from build123d import *

# Parameters (mm, degrees)
SKETCH1_W           = 111.125
SKETCH1_H           = 82.55
SKETCH1_R           = 4.7625
BOSS_EXTRUDE1_DEPTH = 6.35
SKETCH2_R           = 2.413
CUT_EXTRUDE1_DEPTH  = 12.7
SKETCH3_R           = 2.413
CUT_EXTRUDE2_DEPTH  = 12.7
SKETCH4_R           = 2.413
SKETCH4_W           = 22.225
SKETCH4_H           = 22.225
CUT_EXTRUDE3_DEPTH  = 7.62


with BuildPart() as part:
    # Sketch1 → Boss-Extrude1 (new body)
    with BuildSketch(Plane.XY):
        Rectangle(SKETCH1_W, SKETCH1_H)
        with Locations((0, 30.1625)):
            Circle(SKETCH1_R, mode=Mode.SUBTRACT)
        with Locations(Location((0, -30.1625, 0), (0, 0, 180))):
            Circle(SKETCH1_R, mode=Mode.SUBTRACT)
    extrude(amount=BOSS_EXTRUDE1_DEPTH)

    # Sketch2 → Cut-Extrude1 (cut)
    with BuildSketch(Plane(origin=(55.5625, 0, 0), x_dir=(0, 0, -1), z_dir=(1, 0, 0))):
        with Locations((-3.175, 20.6375)):
            Circle(SKETCH2_R)
        with Locations((-3.175, 0)):
            Circle(SKETCH2_R)
        with Locations((-3.175, -20.6375)):
            Circle(SKETCH2_R)
    cut_extrude1 = extrude(amount=-CUT_EXTRUDE1_DEPTH, mode=Mode.SUBTRACT)

    # Mirror1: Cut-Extrude1 across plane
    add(cut_extrude1.mirror(Plane(origin=(0, 0, 0), x_dir=(0, 0, 1), z_dir=(1, 0, 0))), mode=Mode.SUBTRACT)

    # Sketch3 → Cut-Extrude2 (cut)
    with BuildSketch(Plane(origin=(0, 41.275, 0), x_dir=(1, 0, 0), z_dir=(0, 1, 0))):
        with Locations(Location((0, -3.175, 0), (0, 0, 180))):
            Circle(SKETCH3_R)
    cut_extrude2 = extrude(amount=-CUT_EXTRUDE2_DEPTH, mode=Mode.SUBTRACT)

    # Mirror2: Cut-Extrude2 across plane
    add(cut_extrude2.mirror(Plane.ZX), mode=Mode.SUBTRACT)

    # Sketch4 → Cut-Extrude3 (cut)
    with BuildSketch(Plane.XY.offset(6.35)):
        with Locations((17.4625, 0)):
            Circle(SKETCH4_R)
        with Locations((-17.4625, 0)):
            Circle(SKETCH4_R)
        Rectangle(SKETCH4_W, SKETCH4_H)
    extrude(amount=-CUT_EXTRUDE3_DEPTH, mode=Mode.SUBTRACT)


solid = part.part
Source: CAD feature listing. Evaluate the final solid. Frame: model axes, mm. A direction names the side the tool comes from. Give positions to 0.01 mm unless a question says otherwise; leave off trailing zeros. Write each loop counter-clockwise with the first axis right and the second up, starting at its lowest first coordinate (ties: lowest second). Pieces come first, ordered by that corner, then holes. Notation, with made-up numbers: (70.25, -22.75) -> (95.25, -22.75) arc R27 ccw to (95.25, 3.25) -> close; hole circle Ø2 at (-20.75, 88). An arc over 180 degrees is marked (long way). Write item = value, one per line.
Q1. Line query: line 1 (Y direction, x = 6, z = 2) (1 decimal); line 2 (X direction, y = 0.5, z = 1.5); line 3 (Y direction, x = -0.5, z = 5). Output: solid intervals per line, ascending. Write a range as from..to.
Here are the results:
line_1 = -41.3..-11.1, 11.1..41.3
line_2 = -42.86..-19.82, -15.1..-11.11, 11.11..15.1, 19.82..42.86
line_3 = -25.43..-11.11, 11.11..25.43
Q2. Cut plane C-C on y = 19.5. Return loops of the section in (x, z), then the cut area to 3 significant figures.
Here are the results:
outline = (-55.56, 0) -> (55.56, 0) -> (55.56, 1.05) -> (42.86, 1.05) -> (42.86, 5.3) -> (55.56, 5.3) -> (55.56, 6.35) -> (-55.56, 6.35) -> (-55.56, 5.3) -> (-42.86, 5.3) -> (-42.86, 1.05) -> (-55.56, 1.05) -> close
area = 598 mm²
Q3. Mould query, pull axis Z, two halves, no side actions, for faces 1 (the face through (49.301, -19.913, 0.873)), 2 (the face through (42.862, 21, 3)), 3 (the face through (-13, 1, 0)), 4 (the face through (19.764, 0.725, 3.219)). Classes: +Z half, -Z half, draft (parallel to the pull), parting line (faces both ways), or undercut.
Here are the results:
face_1 = undercut
face_2 = undercut
face_3 = -Z half
face_4 = draft
Q4. Reachability of faces 5 (the face through (2.41, -37.82, 3.28)), 6 (the face through (11.112, 0, 3)), 7 (the face through (49.301, -0.924, 0.946)) from +Z, -Z, +X, -X, +Y, -Y: full face, straight path, thin tool, end or side. Return the list, or none.
Here are the results:
face_5 = -Y
face_6 = +Z, -Z
face_7 = +X
Q5. Cut plane A-A on y = -5.5. Return loops of the section in (x, z), then the cut area to 3 significant figures.
Here are the results:
outline = (-55.56, 0) -> (-11.11, 0) -> (-11.11, 6.35) -> (-55.56, 6.35) -> close; (11.11, 0) -> (55.56, 0) -> (55.56, 6.35) -> (11.11, 6.35) -> close
area = 565 mm²
Q6. First-contact query: pin 1 (2.5 mm diameter, centred on y = 20, z = 2.5, fed in from -X); pin 2 (3 mm diameter, centred on x = 0.5, z = 2, fed in from -Y) (3 decimals); pin 3 (2.5 mm diameter, centred on y = -1, z = 3.5, fed in from +X). Flat tips, straight axial feed; report the tip coordinate or a pass-through.
Here are the results:
pin_1 = -42.86
pin_2 = -41.275
pin_3 = 42.86
Q7. Cut plane B-B on x = 0. State how many separate pieces and enclosed holes the cut face has, then the cut area to 3 significant figures.
Here are the results:
separate_pieces = 6
enclosed_holes = 0
area = 201 mm²
